Check sheet for the modelled part. Datum: model origin and axes. Units: mm. Face numbers are marked on the shaded views. A direction names the side the tool comes from. Coordinates: 2 decimals unless noted, no trailing zeros. Loops run counter-clockwise (first coordinate to the right, second up) from the corner with the lowest first, then second, coordinate; pieces in that order, holes last. Notation, with made-up numbers: M 64.5,-12 L 122.5,-12 A25 ccw 122.5,9 Z; hole C 50,-3 d7. An arc over 180 degrees is marked long. Return JSON: item names as keys, results as strings.
from build123d import *

# Parameters (mm, degrees)
EXTRUDE_1_DEPTH            = 5
SKETCH_2_W                 = 20
SKETCH_2_H                 = 20
SKETCH_2_R                 = 1.7
SKETCH_2_H_2               = 5
EXTRUDE_2_DEPTH            = 4.5
MIRROR_2_COPY_1_SKETCH_W   = 20
MIRROR_2_COPY_1_SKETCH_H   = 20
MIRROR_2_COPY_1_SKETCH_R   = 1.7
MIRROR_2_COPY_1_SKETCH_H_2 = 5
MIRROR_2_COPY_1_DEPTH      = 4.5
SKETCH_3_R                 = 45.1
SKETCH_3_R_2               = 32.45
CUT_EXTRUDE_1_DEPTH        = 2
SKETCH_3_3_R               = 1.7
SKETCH_3_3_R_2             = 3.5
CUT_EXTRUDE_2_DEPTH        = 110.111181828
SKETCH_3_4_R               = 10.05
SKETCH_3_4_R_2             = 1.7
CUT_EXTRUDE_3_DEPTH        = 0.5
CUT_EXTRUDE_4_DEPTH        = 110.111181828
FILLET_1_R                 = 4


with BuildPart() as part:
    # Sketch 1 → Extrude 1 (new body)
    with BuildSketch(Plane(origin=(0, 0, 0), x_dir=(1, 0, 0), z_dir=(0, 1, 0))):
        with BuildLine():
            Line((-63, 55), (-63, 35))
            Line((-63, 35), (-55, 35))
            Line((-55, 35), (-46.462183916, 13.526628199))
            ThreePointArc((-46.462183916, 13.526628199), (-31.106656674, -7.145573321), (-7.5, -17.434299833))
            Line((-7.5, -17.434299833), (-7.5, -45))
            Line((-7.5, -45), (-55, -45))
            Line((-55, -45), (-55, -35))
            Line((-55, -35), (-63, -35))
            Line((-63, -35), (-63, -55))
            Line((-63, -55), (63, -55))
            Line((63, -55), (63, -35))
            Line((63, -35), (55, -35))
            Line((55, -35), (55, -45))
            Line((55, -45), (7.5, -45))
            Line((7.5, -45), (7.5, -17.434299833))
            ThreePointArc((7.5, -17.434299833), (31.106656674, -7.145573321), (46.462183916, 13.526628199))
            Line((46.462183916, 13.526628199), (55, 35))
            Line((55, 35), (63, 35))
            Line((63, 35), (63, 55))
            Line((63, 55), (44.395945761, 55))
            ThreePointArc((44.395945761, 55), (0, 82), (-44.395945761, 55))
            Line((-44.395945761, 55), (-63, 55))
        make_face()
    extrude(amount=EXTRUDE_1_DEPTH)

    # Sketch 2 → Extrude 2 (add)
    # profile 1 of 2: a face of its own
    with BuildSketch(Plane(origin=(63, 0, 0), x_dir=(0, 0, -1), z_dir=(1, 0, 0))):
        with Locations((45, -10)):
            Rectangle(SKETCH_2_W, SKETCH_2_H)
        with Locations((45, -16)):
            Circle(SKETCH_2_R, mode=Mode.SUBTRACT)
        with Locations((51, -6)):
            Circle(SKETCH_2_R, mode=Mode.SUBTRACT)
        with Locations((39, -6)):
            Circle(SKETCH_2_R, mode=Mode.SUBTRACT)
    # profile 2 of 2: a face of its own
    with BuildSketch(Plane(origin=(63, 0, 0), x_dir=(0, 0, -1), z_dir=(1, 0, 0))):
        with Locations((45, 2.5)):
            Rectangle(SKETCH_2_W, SKETCH_2_H_2)
    extrude_2 = extrude(amount=EXTRUDE_2_DEPTH)

    # Mirror 1: Extrude 2 across plane
    add(extrude_2.mirror(Plane.XY))

    # Mirror 2: Extrude 2 across plane
    add(extrude_2.mirror(Plane(origin=(0, 0, 0), x_dir=(0, 0, 1), z_dir=(1, 0, 0))))

    # Mirror 2 copy 1 sketch → Mirror 2 copy 1 (add)
    # profile 1 of 2: a face of its own
    with BuildSketch(Plane.ZY.offset(63)):
        with Locations((45, -10)):
            Rectangle(MIRROR_2_COPY_1_SKETCH_W, MIRROR_2_COPY_1_SKETCH_H)
        with Locations((45, -16)):
            Circle(MIRROR_2_COPY_1_SKETCH_R, mode=Mode.SUBTRACT)
        with Locations((51, -6)):
            Circle(MIRROR_2_COPY_1_SKETCH_R, mode=Mode.SUBTRACT)
        with Locations((39, -6)):
            Circle(MIRROR_2_COPY_1_SKETCH_R, mode=Mode.SUBTRACT)
    # profile 2 of 2: a face of its own
    with BuildSketch(Plane.ZY.offset(63)):
        with Locations((45, 2.5)):
            Rectangle(MIRROR_2_COPY_1_SKETCH_W, MIRROR_2_COPY_1_SKETCH_H_2)
    extrude(amount=MIRROR_2_COPY_1_DEPTH)

    # Sketch 3 → Cut-Extrude 1 (cut)
    with BuildSketch(Plane(origin=(0, 5, 0), x_dir=(1, 0, 0), z_dir=(0, 1, 0))):
        with Locations(Location((0, 32, 0), (0, 0, 270))):
            Circle(SKETCH_3_R)
        with Locations(Location((0, 32, 0), (0, 0, 270))):
            Circle(SKETCH_3_R_2, mode=Mode.SUBTRACT)
    extrude(amount=-CUT_EXTRUDE_1_DEPTH, mode=Mode.SUBTRACT)

    # Sketch 3_3 → Cut-Extrude 2 (cut, through all)
    with BuildSketch(Plane(origin=(0, 5, 0), x_dir=(1, 0, 0), z_dir=(0, 1, 0))):
        with Locations(Location((0, 39, 0), (0, 0, 270))):
            Circle(SKETCH_3_3_R)
        with Locations(Location((7, 32, 0), (0, 0, 270))):
            Circle(SKETCH_3_3_R)
        with Locations(Location((0, 25, 0), (0, 0, 270))):
            Circle(SKETCH_3_3_R)
        with Locations(Location((-7, 32, 0), (0, 0, 270))):
            Circle(SKETCH_3_3_R)
        with Locations(Location((0, 32, 0), (0, 0, 270))):
            Circle(SKETCH_3_3_R_2)
    extrude(amount=-CUT_EXTRUDE_2_DEPTH, mode=Mode.SUBTRACT)

    # Sketch 3_4 → Cut-Extrude 3 (cut)
    with BuildSketch(Plane(origin=(0, 5, 0), x_dir=(1, 0, 0), z_dir=(0, 1, 0))):
        with Locations(Location((0, 32, 0), (0, 0, 270))):
            Circle(SKETCH_3_4_R)
        with Locations(Location((-7, 32, 0), (0, 0, 270))):
            Circle(SKETCH_3_4_R_2, mode=Mode.SUBTRACT)
        with Locations(Location((0, 25, 0), (0, 0, 270))):
            Circle(SKETCH_3_4_R_2, mode=Mode.SUBTRACT)
        with Locations(Location((7, 32, 0), (0, 0, 270))):
            Circle(SKETCH_3_4_R_2, mode=Mode.SUBTRACT)
        with Locations(Location((0, 39, 0), (0, 0, 270))):
            Circle(SKETCH_3_4_R_2, mode=Mode.SUBTRACT)
    extrude(amount=-CUT_EXTRUDE_3_DEPTH, mode=Mode.SUBTRACT)

    # Sketch 4 → Cut-Extrude 4 (cut, through all)
    with BuildSketch(Plane(origin=(0, 5, 0), x_dir=(1, 0, 0), z_dir=(0, 1, 0))):
        with BuildLine():
            Line((-18.207999616, 24.398602102), (-11.844038585, 18.034641072))
            ThreePointArc((-11.844038585, 18.034641072), (-8.66205807, 18.034641072), (-8.66205807, 21.216621587))
            Line((-8.66205807, 21.216621587), (-15.0260191, 27.580582618))
            ThreePointArc((-15.0260191, 27.580582618), (-18.207999616, 27.580582618), (-18.207999616, 24.398602102))
        make_face()
    extrude(amount=-CUT_EXTRUDE_4_DEPTH, mode=Mode.SUBTRACT)

    # Fillet 1
    fillet_1_edges = [part.edges().sort_by_distance(p)[0] for p in [
        (-55, 2.5, 35),
        (-55, 2.5, 45),
        (-7.5, 2.5, 45),
        (-7.5, 2.5, 17.434299833),
        (-55, 2.5, -35),
        (-44.395945761, 2.5, -55),
        (44.395945761, 2.5, -55),
        (55, 2.5, -35),
        (7.5, 2.5, 17.434299833),
        (7.5, 2.5, 45),
        (55, 2.5, 45),
        (55, 2.5, 35),
    ]]
    fillet(fillet_1_edges, radius=FILLET_1_R)


solid = part.part
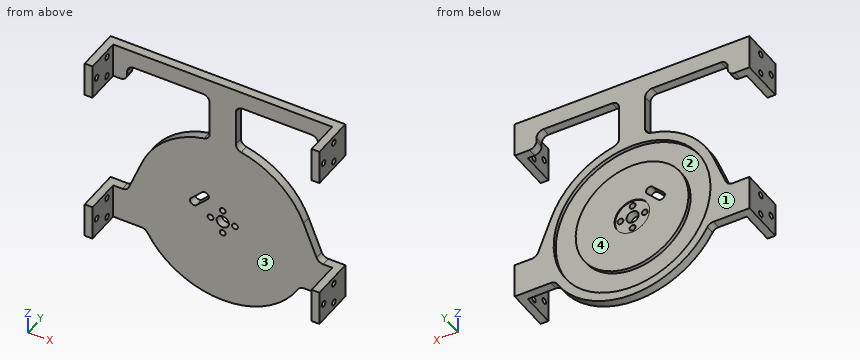
1) Draft check along X on the marked faces 3 and 4. Enter one of: +X half, -X half, draft (parallel to the pull), parting line (faces both ways), or undercut.
Answers:
{"face 3": "undercut", "face 4": "draft"}
2) Section check A-A on x = 0. Record the cut outline in (y, z), then the cut area to 3 significant figures.
Answers:
{"outline": "M 0,-82 L 5,-82 L 5,-77.1 L 3,-77.1 L 3,-64.45 L 5,-64.45 L 5,-42.05 L 4.5,-42.05 L 4.5,-40.7 L 0,-40.7 Z; M 0,-37.3 L 4.5,-37.3 L 4.5,-35.5 L 0,-35.5 Z; M 0,-28.5 L 4.5,-28.5 L 4.5,-26.7 L 0,-26.7 Z; M 0,-23.3 L 4.5,-23.3 L 4.5,-21.95 L 5,-21.95 L 5,0.45 L 3,0.45 L 3,13.1 L 5,13.1 L 5,55 L 0,55 Z", "area": "562 mm²"}
3) Scan lines: line 1 along X through (y, z) = (-12.75, -45); line 2 along Y through (x, z) = (65.85, -39); line 3 along Z through (x, y) = (40, 3.5). Record each from-to range of solid material in increasing order. Write a range as [from, to].
Answers:
{"line 1": "[-67.5, -63], [63, 67.5]", "line 2": "[-20, -7.7], [-4.3, 5]", "line 3": "[-62, -52.83], [-11.17, -2], [45, 55]"}
4) Set-up check for the marked faces 1 and 2: record each of +Z, -Z, +X, -X, +Y, -Y from which the full face is reachable in a straight line by a thin tool's end or side.
Answers:
{"face 1": "+Z, -Z, +X, -X, +Y", "face 2": "+Y"}
5) Section check B-B on z = -45. Record the cut outline in (x, y), then the cut area to 3 significant figures.
Answers:
{"outline": "M -67.5,-20 L -63,-20 L -63,-17.7 L -67.5,-17.7 Z; M -67.5,-14.3 L -63,-14.3 L -63,0 L 63,0 L 63,-14.3 L 67.5,-14.3 L 67.5,5 L 43.19,5 L 43.19,3 L 29.73,3 L 29.73,5 L -29.73,5 L -29.73,3 L -43.19,3 L -43.19,5 L -67.5,5 Z; M 63,-20 L 67.5,-20 L 67.5,-17.7 L 63,-17.7 Z", "area": "771 mm²"}
6) Section check C-C on x = -40. Record the cut outline in (y, z), then the cut area to 3 significant figures.
Answers:
{"outline": "M 0,-62 L 5,-62 L 5,-52.83 L 3,-52.83 L 3,-11.17 L 5,-11.17 L 5,-2 L 0,-2 Z; M 0,45 L 5,45 L 5,55 L 0,55 Z", "area": "267 mm²"}
7) Go/stop test with flat-tipped pins: pin 1 Ø3 at (x, z) = (-9.5, 21) entering from +Y; pin 2 Ø5 at (x, z) = (34.5, -26) entering from +Y; pin 3 Ø4 at (y, z) = (-16, -45) entering from +X; pin 4 Ø12 at (x, z) = (-9, -48.5) entering from -Y. Record where each tip stops, or that it passes through.
Answers:
{"pin 1": "through", "pin 2": "y = 3", "pin 3": "x = 67.5", "pin 4": "y = 0"}
8) Section check D-D on z = -60. Record the cut outline in (x, y), then the cut area to 3 significant figures.
Answers:
{"outline": "M -41.42,0 L 41.42,0 L 41.42,5 L 35.36,5 L 35.36,3 L 16.4,3 L 16.4,5 L -16.4,5 L -16.4,3 L -35.36,3 L -35.36,5 L -41.42,5 Z", "area": "338 mm²"}
